```python
from build123d import *

# Parameters (mm, degrees)
F0_W     = 381
F0_H     = 914.4
F1_DEPTH = 190.5
F2_T     = -2.54
F3_W     = 381
F3_H     = 2.54
F4_DEPTH = 304.8


with BuildPart() as f1:
    # F0 (on Front) → F1 (new body, symmetric)
    with BuildSketch(Plane.XZ):
        Rectangle(F0_W, F0_H)
    extrude(amount=F1_DEPTH, both=True)

    # F2
    f2_openings = [f1.faces().sort_by_distance(p)[0] for p in [
        (0, 0, 457.2),
    ]]
    offset(amount=F2_T, openings=f2_openings)

    # F3 (on face) → F4 (join)
    with BuildSketch(Plane.XY.offset(457.2)):
        with Locations((0, 189.23)):
            Rectangle(F3_W, F3_H)
    extrude(amount=F4_DEPTH)


solid = f1.part
```
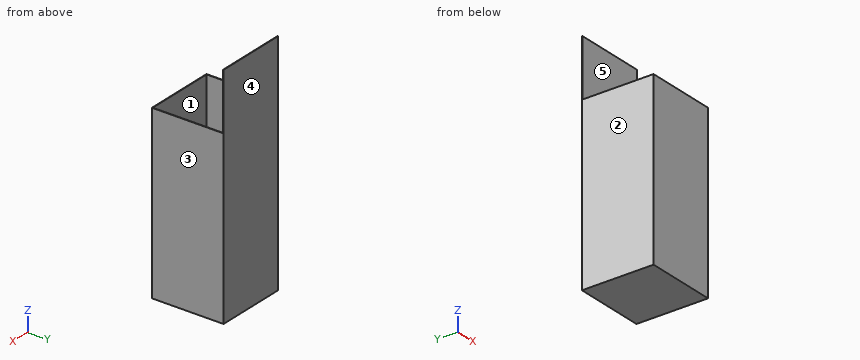
Source: CAD feature listing. Evaluate the final solid. Frame: model axes, mm. Face numbers are marked on the shaded views. A direction names the side the tool comes from. Round coordinates to 2 decimals unless told otherwise and drop trailing zeros. Loops run counter-clockwise (first coordinate to the right, second up) from the corner with the lowest first, then second, coordinate; pieces in that order, holes last. Notation, with made-up numbers: M 51.5,-12 L 77.5,-12 A30 cw 77.5,19 Z; hole C 24.25,48 d1. An arc over 180 degrees is marked long. Use a Markdown table: item, result. Add a question column.
1. Line query: line 1 (Y direction, x = 59.5, z = 65); line 2 (Z direction, x = -128, y = -124). Output: solid intervals per line, ascending.
2. Reachability of the marked faces 4 and 5 from +Z, -Z, +X, -X, +Y, -Y: full face, straight path, thin tool, end or side. Return the list, or none.
3. Section query A-A on x = 54. Return the cut outline in (y, z), then the cut area to 3 significant figures.
4. Mould query, pull axis X, two halves, no side actions, for the marked faces 1, 2 and 3. Classes: pulls with the +X half, pulls with the -X half, needs draft (parallel to the pull), parting line crosses it, or undercut.
5. Section query C-C on y = 109.5. Return the cut outline in (x, z).
6. Section query D-D on z = 687. Return the cut outline in (x, y).
7. Contact query for a flat-ended pin moving along its axis: P1, Ø12, axis at x = 133.5, y = 72.5, coming from the +Z side. Output: stop coordinate, or through.
8. Section query B-B on z = 361.5. Return the cut outline in (x, y), then the cut area to 3 significant figures.
Reported:
| question | item | result |
|---|---|---|
| 1 | line 1 | y = -190.5 to -187.96, 187.96 to 190.5 |
| 1 | line 2 | z = -457.2 to -454.66 |
| 2 | face 4 | +Z, -Z, +X, -X, +Y |
| 2 | face 5 | +Z |
| 3 | outline | M -190.5,-457.2 L 190.5,-457.2 L 190.5,762 L 187.96,762 L 187.96,-454.66 L -187.96,-454.66 L -187.96,457.2 L -190.5,457.2 Z |
| 3 | area | 6,370 mm² |
| 4 | face 1 | undercut |
| 4 | face 2 | pulls with the -X half |
| 4 | face 3 | pulls with the +X half |
| 5 | outline | M -190.5,-457.2 L 190.5,-457.2 L 190.5,457.2 L 187.96,457.2 L 187.96,-454.66 L -187.96,-454.66 L -187.96,457.2 L -190.5,457.2 Z |
| 6 | outline | M -190.5,187.96 L 190.5,187.96 L 190.5,190.5 L -190.5,190.5 Z |
| 7 | P1 | stops at z = -454.66 |
| 8 | outline | M -190.5,-190.5 L 190.5,-190.5 L 190.5,190.5 L -190.5,190.5 Z; hole M -187.96,-187.96 L 187.96,-187.96 L 187.96,187.96 L -187.96,187.96 Z |
| 8 | area | 3,850 mm² |
